Input: part model. Units: mm. Frame: model coordinates. Round coordinates to 2 decimals unless told otherwise and drop trailing zeros. Loops run counter-clockwise (first coordinate to the right, second up) from the corner with the lowest first, then second, coordinate; pieces in that order, holes last. Notation, with made-up numbers: M 80,8.5 L 97,8.5 A22 cw 97,22.5 Z; hole C 53.25,61.5 d10. An arc over 180 degrees is marked long. Return JSON: item names as keys, results as strings. Group by question number.
1) Section C-C (y = -37). Output: boundary loops of the cut face in (x, z).
2) Material intervals for line 1 (X direction, y = -12.25, z = 0); line 2 (Y direction, x = 0, z = 10.5), sorted ascending. Write a range as from..to.
3) Contact query for flat-ended pins moving along their axis: P1, Ø3, axis at y = -1, z = -8, coming from the +X side; P2, Ø1, axis at y = -236, z = -2.5, coming from the +X side; P3, Ø0.8, axis at y = -1.5, z = 8.5, coming from the -X side; P4, Ø4.5, axis at x = 9, z = -1, coming from the +Y side. Output: stop coordinate, or through.
4) Section B-B (z = 0). Output: boundary loops of the cut face in (x, y), plus the area to 3 significant figures.
5) Section A-A (x = 0). Output: boundary loops of the cut face in (y, z), plus the area to 3 significant figures.
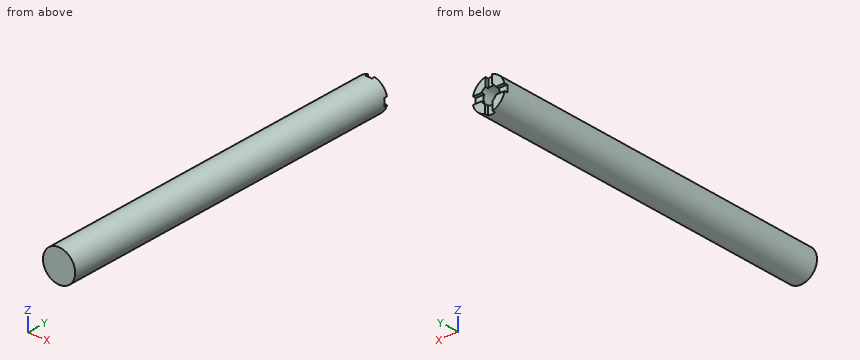
from build123d import *

# Parameters (mm, degrees)
F0_R     = 12.7
F1_DEPTH = 279.4
F2_R     = 6.35
F3_DEPTH = 19.05
F4_W     = 5.08
F4_H     = 10.381874
F4_W_2   = 11.262799
F4_H_2   = 5.378819
F4_W_3   = 5.677644
F4_H_3   = 9.531256
F4_W_4   = 10.833798
F4_H_4   = 5.677642
F5_DEPTH = 2.54


with BuildPart() as f1:
    # F0 (on Front) → F1 (new body)
    with BuildSketch(Plane.XZ):
        Circle(F0_R)
    extrude(amount=F1_DEPTH)

    # F2 (on face) → F3 (cut)
    with BuildSketch(Plane(origin=(0, 0, 0), x_dir=(-1, 0, 0), z_dir=(0, 1, 0))):
        Circle(F2_R)
    extrude(amount=-F3_DEPTH, mode=Mode.SUBTRACT)

    # F4 (on Front) → F5 (cut)
    with BuildSketch(Plane.XZ):
        with Locations((0.023213, 10.806244)):
            Rectangle(F4_W, F4_H)
        with Locations((-10.631255, 0.159545)):
            Rectangle(F4_W_2, F4_H_2)
        with Locations((0.023213, -9.717169)):
            Rectangle(F4_W_3, F4_H_3)
        with Locations((10.593361, 0.010134)):
            Rectangle(F4_W_4, F4_H_4)
    extrude(amount=F5_DEPTH, mode=Mode.SUBTRACT)


solid = f1.part
Returned:
{
 "1": {"outline": "C 0,0 d25.4"},
 "2": {"line 1": "x = -12.7..-6.35, 6.35..12.7", "line 2": "y = -279.4..-2.54"},
 "3": {"P1": "stops at x = 10.91", "P2": "stops at x = 12.54", "P3": "stops at x = -9.78", "P4": "stops at y = 0"},
 "4": {"outline": "M -12.7,-279.4 L 12.7,-279.4 L 12.7,-2.54 L 6.35,-2.54 L 6.35,-19.05 L -6.35,-19.05 L -6.35,-2.54 L -12.7,-2.54 Z", "area": "6,820 mm^2"},
 "5": {"outline": "M -279.4,-12.7 L -2.54,-12.7 L -2.54,-6.35 L -19.05,-6.35 L -19.05,6.35 L -2.54,6.35 L -2.54,12.7 L -279.4,12.7 Z", "area": "6,820 mm^2"}
}
